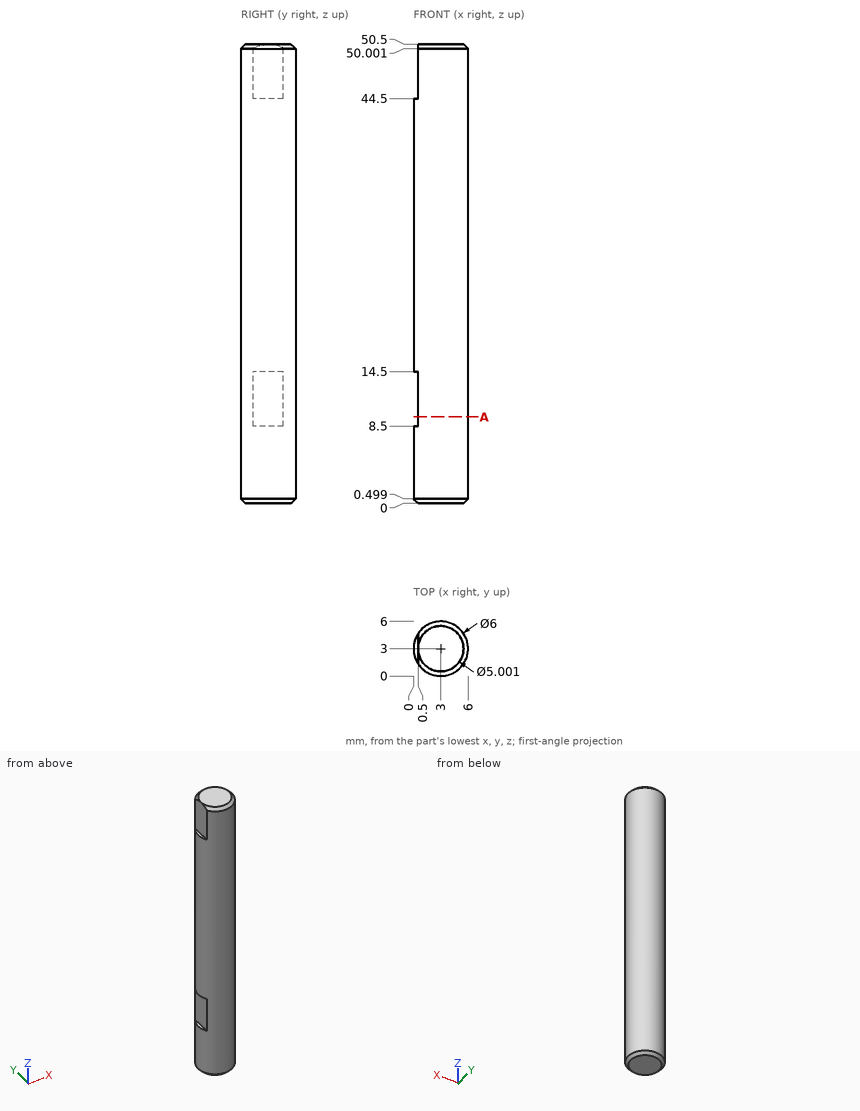
Source: three-view drawing plus pictorial views. Frame: mm from the lowest corner of the part. Coordinates: 2 decimals unless noted, no trailing zeros. Order: outer loops, then holes, each group sorted by start corner. A loop starts at its lowest first (then second) coordinate and runs counter-clockwise, first axis right, second up. Notation, with made-up numbers: (73, -21) -> (88, -21) arc R22 cw to (88, 13) -> close; hole circle Ø7 at (-38, 36.25). An arc over 180 degrees is marked (long way). Write item = value, one per line.
(1) Line query: line 1 (Y direction, x = 2.9, z = 18.5); line 2 (Z direction, x = 4.45, y = 5.1); line 3 (X direction, y = 1.55, z = 6) (1 decimal). Output: solid intervals per line, ascending.
Solved:
line_1 = 0 to 6
line_2 = 0.05 to 50.45
line_3 = 0.4 to 5.6
(2) Pin query (flat end, axial travel): pin 1 Ø2.5 at (y, z) = (3.5, 47.5) entering from -X. Return the tip coordinate at first contact, or that it passes through.
Solved:
pin_1 = 0.5
(3) Cut plane A-A on z = 9.5. Return loops of the section in (x, y).
Solved:
outline = (0.5, 1.34) arc R3 ccw (long way) to (0.5, 4.66) -> close
